Here's the drawing with two shaded views (mm, measured from the low corner). I have some questions. Give positions to 0.01 mm unless a question says otherwise; leave off trailing zeros. Loops run counter-clockwise (first coordinate to the right, second up) from the corner with the lowest first, then second, coordinate; pieces in that order, holes last. Notation, with made-up numbers: (27, 13.5) -> (71, 13.5) arc R6 cw to (71, 21.5) -> close; hole circle Ø7 at (28.25, 23.25). An arc over 180 degrees is marked (long way). Answer in a Markdown table with one row per item. Add a question column.
Item 1: If we section it at A-A (x = 7.5): Give the number of separate pieces and of enclosed holes in the cut face, then the cut area to 3 significant figures.
Item 2: If we section it at C-C (x = 66.5): Write out the boundary of the cut face in (y, z) (1 decimal), then the cut area to 3 significant figures.
Item 3: If I drill on line 1 (Y direction, x = 64, z = 2.1) (1 decimal); line 2 (X direction, y = 57, z = 0.7) (1 decimal); line 3 (X direction, y = 56, z = 1) (1 decimal), over which ranges is the centre line in solid material (lowest first)?
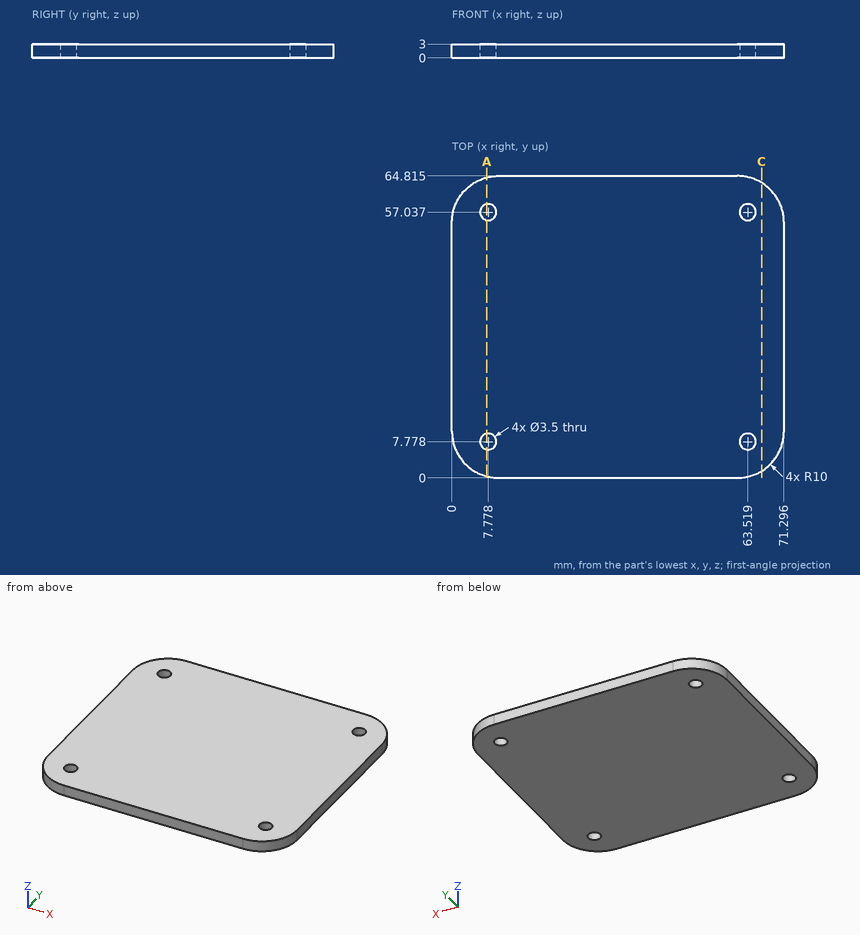
Recorded:
| question | item | result |
|---|---|---|
| 1 | separate pieces | 3 |
| 1 | enclosed holes | 0 |
| 1 | area | 172 mm^2 |
| 2 | outline | (1.5, 0) -> (63.4, 0) -> (63.4, 3) -> (1.5, 3) -> close |
| 2 | area | 186 mm^2 |
| 3 | line 1 | y = 0.4 to 6.1, 9.5 to 55.4, 58.7 to 64.4 |
| 3 | line 2 | x = 0.2 to 6, 9.5 to 61.8, 65.3 to 71.1 |
| 3 | line 3 | x = 0.1 to 6.4, 9.2 to 62.1, 64.9 to 71.2 |
